Could you check a few things on this model? Use its own coordinates, in mm. Face numbers are marked on the shaded views. A direction names the side the tool comes from. Coordinates: 2 decimals unless noted, no trailing zeros. Loops run counter-clockwise (first coordinate to the right, second up) from the corner with the lowest first, then second, coordinate; pieces in that order, holes last. Notation, with made-up numbers: M 0.5,64.25 L 28.5,64.25 A28 ccw 28.5,85.25 Z; hole C 6.5,34.25 d3. An arc over 180 degrees is marked long. Write each question's results on one line, items separated by ' | '.
```python
from build123d import *

# Parameters (mm, degrees)
SKETCH1_W = 1.5
SKETCH1_H = 3


with BuildPart() as part:
    # Sketch1 → Revolve1 (revolve)
    with BuildSketch(Plane(origin=(0, 0, 0), x_dir=(0, 0, -1), z_dir=(1, 0, 0)), mode=Mode.PRIVATE) as revolve1_sk:
        Polygon((10.5, 6), (0, 6), (0, 3), (3, 3), (4.5, 3), (10.5, 3), align=None)
        with Locations((3.75, 1.5)):
            Rectangle(SKETCH1_W, SKETCH1_H)
    revolve(revolve1_sk.sketch.rotate(Axis((0, 0, 0), (0, -1, 0)), 180), axis=Axis((0, 0, 0), (0, -1, 0)))


solid = part.part
```
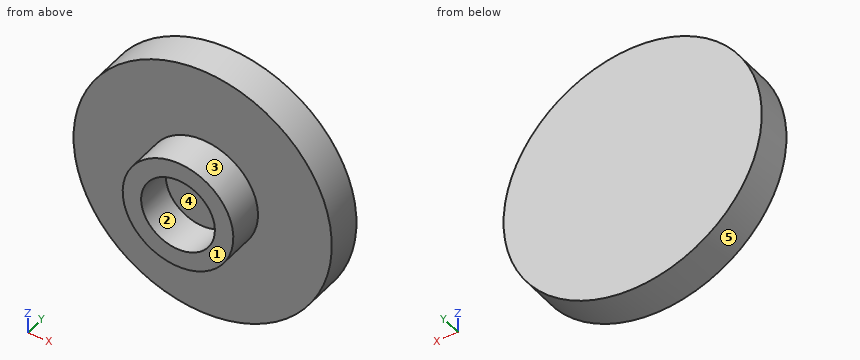
(1) Will these pins go through, and if not, where does the flat tip stop? P1, Ø2, axis at x = -2, y = 3, coming from the +Z side; P2, Ø1.8, axis at x = -0.5, z = 0, coming from the -Y side; P3, Ø2, axis at x = -1.5, y = 4.5, coming from the -Z side.
Reported:
P1: stops at z = 10.45 | P2: stops at y = 3 | P3: stops at z = -10.49
(2) Imagine slicing it at A-A, the plane z = 0. List the corners of the cut face in (x, y) for me, and give its area (3 significant figures).
Reported:
outline: M -10.5,3 L -4.5,3 L -4.5,0 L -3,0 L -3,3 L 3,3 L 3,0 L 4.5,0 L 4.5,3 L 10.5,3 L 10.5,6 L -10.5,6 Z | area: 72.0 mm2
(3) Imagine slicing it at C-C, the plane y = 0.45. List the corners of the cut face in (x, z) for me.
Reported:
outline: C 0,0 d9; hole C 0,0 d6
(4) Please list where these lines run through material, in increasing order: probe 1 along X at (y, z) = (2.15, 0); probe 2 along Y at (x, z) = (-9.25, -1.5); probe 3 along X at (y, z) = (2.4, -0.75). Write a range as from..to.
Reported:
probe 1: x = -4.5..-3, 3..4.5 | probe 2: y = 3..6 | probe 3: x = -4.44..-2.9, 2.9..4.44
(5) If we mould it in two halves opening along Z, with no side actions, what happens to the marked faces 1, 2 and 3? For each: released by +Z, released by -Z, zero draft, split by the parting line, or undercut.
Reported:
face 1: zero draft | face 2: undercut | face 3: split by the parting line
(6) Which directions (+Z, -Z, +X, -X, +Y, -Y) give clear straight access to the entire face, cutting with the end or side of a thin tool? Please do the marked faces 4 and 5.
Reported:
face 4: -Y | face 5: +Y, -Y
(7) Imagine slicing it at B-B, the plane x = 0. List the corners of the cut face in (y, z) for me.
Reported:
outline: M 0,-4.5 L 3,-4.5 L 3,-10.5 L 6,-10.5 L 6,10.5 L 3,10.5 L 3,4.5 L 0,4.5 L 0,3 L 3,3 L 3,-3 L 0,-3 Z
(8) Imagine slicing it at D-D, the plane y = 4.35. List the corners of the cut face in (x, z) for me, and give its area (3 significant figures).
Reported:
outline: C 0,0 d21 | area: 346 mm2
